Read the model definition and answer for the solid it produces. Units are mm, in the model's axes. Face numbers are marked on the shaded views. A direction names the side the tool comes from. Give positions to 0.01 mm unless a question says otherwise; leave off trailing zeros. Order: outer loops, then holes, each group sorted by start corner. A loop starts at its lowest first (then second) coordinate and runs counter-clockwise, first axis right, second up. Notation, with made-up numbers: (-28, 27) -> (25, 27) arc R13 cw to (25, 52) -> close; hole circle Ø9 at (33, 18.5). An arc over 180 degrees is marked (long way). One line per question, with ' | ' between items. Start each with the question number.
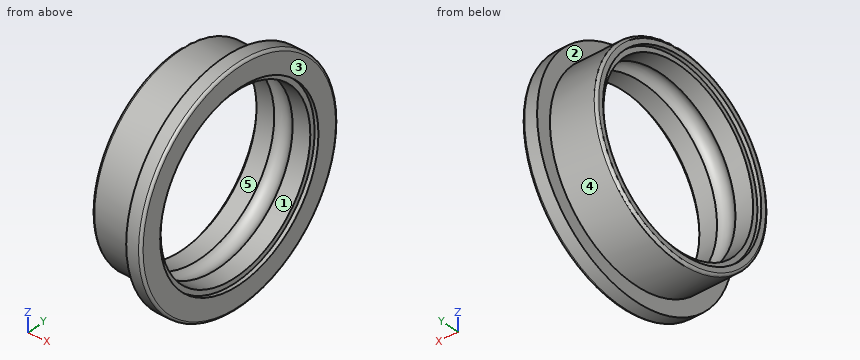
Autodesk Inventor part; units mm, degrees
ref_plane "ip_st_1_XY" through (0, 0, 0) normal (1, 0, 0) x (0, 0, -1)
ref_plane "ip_st_1_YZ" through (0, 0, 0) normal (0, 0, -1) x (0, 1, 0)
ref_plane "ip_st_1_ZX" through (0, 0, 0) normal (0, 1, 0) x (1, 0, 0)
sketch "Sketch_1" plane through (0, 0, 0) normal (0, 0, 1) x (1, 0, 0)
  line L0 (2.5, 0) -> (0, 0)
  line L1 (0, 3.7) -> (0.1562, 3.7)
  line L2 (0.1562, 3.7) -> (0.1562, 3.5)
  line L3 (0.1562, 3.5) -> (0.8758, 3.5)
  arc A0 (1.6242, 3.5) -> (0.8758, 3.5) centre (1.25, 3.25) ccw
  line L4 (1.6242, 3.5) -> (2.3438, 3.5)
  line L5 (2.3438, 3.5) -> (2.3438, 3.7)
  line L6 (2.3438, 3.7) -> (2.5, 3.7)
  line L7 (2.5, 3.7) -> (2.5, 4.5)
  arc A1 (2.5, 4.5) -> (2.4, 4.6) centre (2.4, 4.5) ccw
  line L8 (2.4, 4.6) -> (1.9, 4.6)
  line L9 (1.9, 4.6) -> (1.9, 4)
  line L10 (1.9, 4) -> (0.1, 4)
  arc A2 (0.1, 4) -> (0, 3.9) centre (0.1, 3.9) ccw
  line L11 (0, 3.9) -> (0, 3.7)
revolve "Revolution1" add sketch "Sketch_1" angle 360 about axis through (2.5, 0, 0) along (1, 0, 0)
ref_plane "ip_st_1_XY" through (0, 0, 0) normal (1, 0, 0) x (0, 0, -1)
ref_plane "ip_st_1_YZ" through (0, 0, 0) normal (0, 0, -1) x (0, 1, 0)
ref_plane "ip_st_1_ZX" through (0, 0, 0) normal (0, 1, 0) x (1, 0, 0)
ref_plane "ip_st_2_XY" through (2.3438, 0, 0) normal (-1, 0, 0) x (0, 0, -1)
ref_plane "ip_st_2_YZ" through (2.3438, 0, 0) normal (0, 0, -1) x (0, -1, 0)
ref_plane "ip_st_2_ZX" through (2.3438, 0, 0) normal (0, -1, 0) x (-1, 0, 0)
properties part number "MF85ZZ Outer Ring" material "ステンレス鋼 440C"
Q1. Find the intervals of material crossed by line 1 (Z direction, x = 0.35, y = 0); line 2 (Y direction, x = 0.85, z = 0.5); line 3 (X direction, y = 2.5, z = -3.75), in increasing order.
Q2. A cutting plane is placed at A-A, the plane y = 0. Determine the outline of the cut face in (x, z).
Q3. A cutting plane is placed at C-C, the plane x = 1.5. Determine the outline of the cut face in (y, z), then the cut area to 3 significant figures.
Q4. Determine the mould class of the marked faces 3, 4 and 5 for opening direction Z: pulls with the +Z half, pulls with the -Z half, needs draft (parallel to the pull), parting line crosses it, or undercut.
Q5. Which of the six approach directions +Z, -Z, +X, -X, +Y, -Y give full straight-line access (tool end or side, diameter ignored) to the marked faces 1 and 2?
Q6. Given P1, Ø1.5, axis at x = 1, y = -3, coming from the -Z side; P2, Ø5.5, axis at y = 0, z = 0, coming from the -X side; P3, Ø1.5, axis at x = 2, z = 2.5, coming from the -Y side, each flat-ended and moving along its own axis, determine where each tip first touches the part or whether it passes through.
Geometry results:
1) line 1: -4 to -3.5, 3.5 to 4 | line 2: -3.97 to -3.46, 3.46 to 3.97 | line 3: 1.9 to 2.5
2) outline: (0, -3.9) arc R0.1 ccw to (0.1, -4) -> (1.9, -4) -> (1.9, -4.6) -> (2.4, -4.6) arc R0.1 ccw to (2.5, -4.5) -> (2.5, -3.7) -> (2.34, -3.7) -> (2.34, -3.5) -> (1.62, -3.5) arc R0.45 cw to (0.88, -3.5) -> (0.16, -3.5) -> (0.16, -3.7) -> (0, -3.7) -> close; (0, 3.7) -> (0.16, 3.7) -> (0.16, 3.5) -> (0.88, 3.5) arc R0.45 cw to (1.62, 3.5) -> (2.34, 3.5) -> (2.34, 3.7) -> (2.5, 3.7) -> (2.5, 4.5) arc R0.1 ccw to (2.4, 4.6) -> (1.9, 4.6) -> (1.9, 4) -> (0.1, 4) arc R0.1 ccw to (0, 3.9) -> close
3) outline: circle Ø8 at (0, 0); hole circle Ø7.25 at (0, 0) | area: 9.00 mm²
4) face 3: needs draft | face 4: parting line crosses it | face 5: undercut
5) face 1: +X, -X | face 2: -X
6) P1: z = -3.31 | P2: through | P3: y = -4.25
